Geometry check sheet. Reference: the model listing, model coordinates, mm. Give positions to 0.01 mm unless a question says otherwise; leave off trailing zeros. Write each loop counter-clockwise with the first axis right and the second up, starting at its lowest first coordinate (ties: lowest second). Pieces come first, ordered by that corner, then holes. Notation, with made-up numbers: M 32,-32.5 L 58,-32.5 A22 ccw 58,-12.5 Z; hole C -27.5,-26 d10. An arc over 180 degrees is marked long. Use one line per item in the form item = value. Start each with the question number.
```python
from build123d import *

# Parameters (mm, degrees)
SKETCH1_R           = 1.55
BOSS_EXTRUDE1_DEPTH = 3
SKETCH2_R           = 3.75
CUT_EXTRUDE1_DEPTH  = 3


with BuildPart() as part:
    # Sketch1 → Boss-Extrude1 (new body)
    with BuildSketch(Plane(origin=(0, 0, 0), x_dir=(1, 0, 0), z_dir=(0, 1, 0))):
        with BuildLine():
            Line((0, 0), (94, 0))
            ThreePointArc((94, 0), (47, 47), (0, 0))
        make_face()
        with Locations((47, 3)):
            Circle(SKETCH1_R, mode=Mode.SUBTRACT)
    extrude(amount=BOSS_EXTRUDE1_DEPTH)

    # Sketch2 → Cut-Extrude1 (cut)
    with BuildSketch(Plane(origin=(0, 3, 0), x_dir=(1, 0, 0), z_dir=(0, 1, 0))):
        with Locations((47, 18)):
            Circle(SKETCH2_R)
        with Locations((32, 18)):
            Circle(SKETCH2_R)
        with Locations((62, 18)):
            Circle(SKETCH2_R)
    extrude(amount=-CUT_EXTRUDE1_DEPTH, mode=Mode.SUBTRACT)


solid = part.part
```
(1) Sectioned sample at C-C, the plane y = 0.55. Record the boundary of the cut face in (x, z), plus the area to 3 significant figures.
(2) Sectioned sample at A-A, the plane x = 47. Record the boundary of the cut face in (y, z).
(3) Thickness scan on probe 1 along Z at (x, y) = (47, 2.2); probe 2 along X at (y, z) = (1.9, -18); probe 3 along X at (y, z) = (1.65, -21). Record the ranges inside material, lowest first. Write a range as [from, to].
(4) Sectioned sample at D-D, the plane z = -3. Record the boundary of the cut face in (x, y), plus the area to 3 significant figures.
(5) Draft check along Z on faces 1 (the flat face through (46, 0, -24)), 2 (the cylindrical face through (48.03, 1.48, -46.99)), 3 (the cylindrical face through (48.478, 1.479, -3.466)). Enter one of: released by +Z, released by -Z, zero draft, split by the parting line, or undercut.
(6) Sectioned sample at B-B, the plane z = -18. Record the boundary of the cut face in (x, y).
(7) Depth check by flat-ended pin: pin 1 (4.5 mm diameter, centred on x = 47, z = -18, fed in from +Y); pin 2 (1 mm diameter, centred on y = 1, z = -31, fed in from +X); pin 3 (1.5 mm diameter, centred on y = 0.5, z = -26.5, fed in from +X); pin 4 (4 mm diameter, centred on x = 47, z = -3, fed in from -Y). Enter the tip coordinate at first touch or a pass-through.
Numbers:
q1.outline = M 0,0 A47 ccw 94,0 Z; hole C 32,-18 d7.5; hole C 47,-18 d7.5; hole C 47,-3 d3.1; hole C 62,-18 d7.5
q1.area = 3,330 mm2
q2.outline = M 0,-47 L 3,-47 L 3,-21.75 L 0,-21.75 Z; M 0,-14.25 L 3,-14.25 L 3,-4.55 L 0,-4.55 Z; M 0,-1.45 L 3,-1.45 L 3,0 L 0,0 Z
q3.probe_1 = [-47, -21.75], [-14.25, -4.55], [-1.45, 0]
q3.probe_2 = [3.58, 28.25], [35.75, 43.25], [50.75, 58.25], [65.75, 90.42]
q3.probe_3 = [4.95, 29.75], [34.25, 44.75], [49.25, 59.75], [64.25, 89.05]
q4.outline = M 0.1,0 L 45.45,0 L 45.45,3 L 0.1,3 Z; M 48.55,0 L 93.9,0 L 93.9,3 L 48.55,3 Z
q4.area = 272 mm2
q5.face_1 = zero draft
q5.face_2 = released by -Z
q5.face_3 = undercut
q6.outline = M 3.58,0 L 28.25,0 L 28.25,3 L 3.58,3 Z; M 35.75,0 L 43.25,0 L 43.25,3 L 35.75,3 Z; M 50.75,0 L 58.25,0 L 58.25,3 L 50.75,3 Z; M 65.75,0 L 90.42,0 L 90.42,3 L 65.75,3 Z
q7.pin_1 = through
q7.pin_2 = 82.76
q7.pin_3 = 86.32
q7.pin_4 = 0
